from build123d import *

# Parameters (mm, degrees)
SKETCH1_W           = 167.5
SKETCH1_H           = 50
BOSS_EXTRUDE1_DEPTH = 5
BOSS_EXTRUDE2_REACH = 125.711
SKETCH3_R           = 2
CUT_EXTRUDE1_DEPTH  = 125.190739079
SKETCH6_R           = 1.947134786
BOSS_EXTRUDE7_DEPTH = 2.5
BOSS_EXTRUDE9_REACH = 133.18
SKETCH10_R          = 2
CUT_EXTRUDE3_DEPTH  = 132.180305898
FILLET2_R           = 5
SKETCH11_W          = 132.04
SKETCH11_H          = 9.88782449
CUT_EXTRUDE5_DEPTH  = 36


with BuildPart() as part:
    # Sketch1 → Boss-Extrude1 (new body)
    with BuildSketch(Plane.XY):
        Polygon((-83.75, 30), (-83.75, 55), (-89.745973018, 55), (-89.745973018, -55), (-83.75, -55), (-83.75, -30), (83.75, -30), (83.75, -55), (89.745973018, -55), (89.745973018, 55), (83.75, 55), (83.75, 30), align=None)
        Rectangle(SKETCH1_W, SKETCH1_H, mode=Mode.SUBTRACT)
    extrude(amount=BOSS_EXTRUDE1_DEPTH)

    # Boss-Extrude2: up to this face of the body (flat: up to its plane)
    boss_extrude2_end = Plane(part.part.faces().sort_by_distance((0, -30, 2.5))[0])
    # Sketch2 → Boss-Extrude2 (add, up to the picked face)
    with BuildSketch(Plane(origin=(0, 30, 0), x_dir=(1, 0, 0), z_dir=(0, 1, 0)), mode=Mode.PRIVATE) as boss_extrude2_sk1:
        with BuildLine():
            Line((-56.79, -5), (-63.79, -5))
            ThreePointArc((-63.79, -5), (-56.79, -12), (-49.79, -5))
            Line((-49.79, -5), (-56.79, -5))
        make_face()
    boss_extrude2_tool1 = split(extrude(boss_extrude2_sk1.sketch, amount=-BOSS_EXTRUDE2_REACH, mode=Mode.PRIVATE), bisect_by=boss_extrude2_end, keep=Keep.BOTH, mode=Mode.PRIVATE)
    # Sketch2 → Boss-Extrude2 (add, up to the picked face)
    with BuildSketch(Plane(origin=(0, 30, 0), x_dir=(1, 0, 0), z_dir=(0, 1, 0)), mode=Mode.PRIVATE) as boss_extrude2_sk2:
        Polygon((-63.79, 0), (-63.79, -5), (-56.79, -5), (-49.79, -5), (-49.79, 0), align=None)
    boss_extrude2_tool2 = split(extrude(boss_extrude2_sk2.sketch, amount=-BOSS_EXTRUDE2_REACH, mode=Mode.PRIVATE), bisect_by=boss_extrude2_end, keep=Keep.BOTH, mode=Mode.PRIVATE)
    add(boss_extrude2_tool1.solids().sort_by(Axis((-56.79, 30, 7.970892), (0, -1, 0)))[0])
    add(boss_extrude2_tool2.solids().sort_by(Axis((-56.79, 30, 2.5), (0, -1, 0)))[0])

    # Sketch3 → Cut-Extrude1 (cut, through all)
    with BuildSketch(Plane(origin=(0, 30, 0), x_dir=(1, 0, 0), z_dir=(0, 1, 0))):
        with Locations(Location((-56.79, -5, 0), (0, 0, 270))):
            Circle(SKETCH3_R)
    extrude(amount=-CUT_EXTRUDE1_DEPTH, mode=Mode.SUBTRACT)



with BuildPart() as body_2:
    # Sketch6 → Revolve2 (revolve)
    with BuildSketch(Plane(origin=(0, 0, 0), x_dir=(1, 0, 0), z_dir=(0, 1, 0))):
        with Locations((-97.245973018, -1.947134786)):
            Circle(SKETCH6_R)
    revolve(axis=Axis((-94.745973018, 0, 0), (0, 0, 1)))


with BuildPart() as part_1:
    add(part.part)

    add(body_2.part)  # Boss-Extrude7 merges body 2
    # Sketch9 → Boss-Extrude7 (add, symmetric)
    with BuildSketch(Plane(origin=(0, 0, 0), x_dir=(1, 0, 0), z_dir=(0, 1, 0))):
        Polygon((-92.245973018, 0), (-89.745973018, 0), (-89.745973018, -5), align=None)
    extrude(amount=BOSS_EXTRUDE7_DEPTH, both=True)

    # Boss-Extrude9: up to this face of the body (flat: up to its plane)
    boss_extrude9_end = Plane(part_1.part.faces().sort_by_distance((-4.055234189, -30, 2.93205693))[0])
    # Sketch4 → Boss-Extrude9 (add, up to the picked face)
    with BuildSketch(Plane(origin=(0, 30, 0), x_dir=(1, 0, 0), z_dir=(0, 1, 0)), mode=Mode.PRIVATE) as boss_extrude9_sk1:
        with BuildLine():
            Line((68.25, 0), (68.25, -5))
            ThreePointArc((68.25, -5), (61.25, -12), (54.25, -5))
            Line((54.25, -5), (54.25, 0))
            Line((54.25, 0), (68.25, 0))
        make_face()
    boss_extrude9_tool1 = split(extrude(boss_extrude9_sk1.sketch, amount=-BOSS_EXTRUDE9_REACH, mode=Mode.PRIVATE), bisect_by=boss_extrude9_end, keep=Keep.BOTH, mode=Mode.PRIVATE)
    add(boss_extrude9_tool1.solids().sort_by(Axis((61.25, 30, 5.365156), (0, -1, 0)))[0])

    # Sketch10 → Cut-Extrude3 (cut, through all)
    with BuildSketch(Plane(origin=(0, 30, 0), x_dir=(1, 0, 0), z_dir=(0, 1, 0))):
        with Locations(Location((61.25, -5, 0), (0, 0, 270))):
            Circle(SKETCH10_R)
    extrude(amount=-CUT_EXTRUDE3_DEPTH, mode=Mode.SUBTRACT)

    # Fillet2
    fillet2_edges = [part_1.edges().sort_by_distance(p)[0] for p in [
        (89.745973018, -55, 2.5),
        (89.745973018, 55, 2.5),
        (-89.745973018, 55, 2.5),
        (-89.745973018, -55, 2.5),
    ]]
    fillet(fillet2_edges, radius=FILLET2_R)

    # Sketch11 → Cut-Extrude5 (cut)
    with BuildSketch(Plane(origin=(0, 0, 0), x_dir=(-1, 0, 0), z_dir=(0, 0, -1))):
        with Locations((-2.23, 0)):
            Rectangle(SKETCH11_W, SKETCH11_H)
    extrude(amount=-CUT_EXTRUDE5_DEPTH, mode=Mode.SUBTRACT)


solid = part_1.part
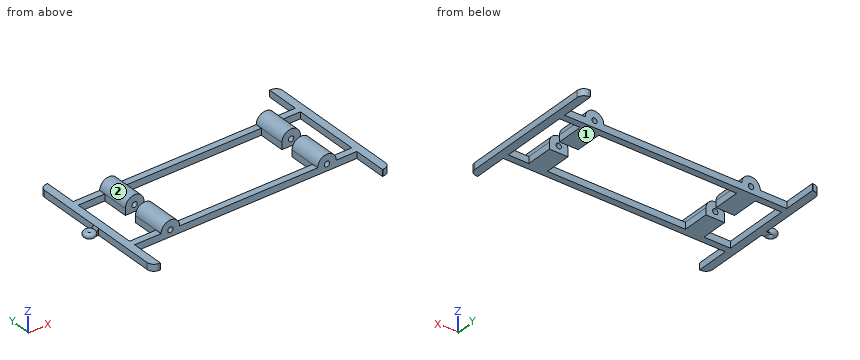
Work out the finished part from the listing and answer in its coordinate system (mm). Face numbers are marked on the shaded views. Round coordinates to 2 decimals unless told otherwise and drop trailing zeros. Write each loop counter-clockwise with the first axis right and the second up, starting at its lowest first coordinate (ties: lowest second). Pieces come first, ordered by that corner, then holes. Notation, with made-up numbers: (-7, 33) - (1, 33) arc R29 ccw to (1, 65) - close; hole circle Ø6 at (84, 81). An arc over 180 degrees is marked (long way). Answer in a Markdown table with one row per item. Add a question column.
1. The mould has two halves that part along X. Classify the marked faces 1 and 2: +X half, -X half, draft (parallel to the pull), parting line (faces both ways), or undercut.
2. A cutting plane is placed at A-A, the plane y = 44.5. Determine the outline of the cut face in (x, z), and give its area (3 significant figures).
3. A cutting plane is placed at B-B, the plane x = 61.25. Determine the outline of the cut face in (y, z).
4. A cutting plane is placed at C-C, the plane z = 9.5. Determine the outline of the cut face in (x, y), and give its area (3 significant figures).
5. Given pin 1 (1.3 mm diameter, centred on x = -91.5, z = 3, fed in from +Y); pin 2 (2.5 mm diameter, centred on y = 13.5, z = 3.5, fed in from -X); pin 3 (1.5 mm diameter, centred on x = -69.5, z = 2.5, fed in from -Y); pin 4 (4 mm diameter, centred on y = -40, z = 7.5, fed in from -X), each flat-ended and moving along its own axis, determine where each tip first touches the part or whether it passes through.
6. Find the intervals of material crossed by line 1 along X through (y, z) = (-27, 5.25); line 2 along X through (y, z) = (-38.5, 1); line 3 along Y through (x, z) = (-74.5, 4.5), in increasing order. Write a range as from..to.
7. A cutting plane is placed at D-D, the plane x = -11. Determine the outline of the cut face in (y, z), and give its area (3 significant figures).
Worked out:
| question | item | result |
|---|---|---|
| 1 | face 1 | draft |
| 1 | face 2 | undercut |
| 2 | outline | (-89.75, 0) - (-83.75, 0) - (-83.75, 5) - (-89.75, 5) - close; (83.75, 0) - (89.75, 0) - (89.75, 5) - (83.75, 5) - close |
| 2 | area | 60.0 mm^2 |
| 3 | outline | (-30, 0) - (-4.94, 0) - (-4.94, 3) - (-30, 3) - close; (-30, 7) - (-4.94, 7) - (-4.94, 12) - (-30, 12) - close; (4.94, 0) - (30, 0) - (30, 3) - (4.94, 3) - close; (4.94, 7) - (30, 7) - (30, 12) - (4.94, 12) - close |
| 4 | outline | (-62.15, -30) - (-51.43, -30) - (-51.43, -4.94) - (-62.15, -4.94) - close; (-62.15, 4.94) - (-51.43, 4.94) - (-51.43, 30) - (-62.15, 30) - close; (55.89, -30) - (66.61, -30) - (66.61, -4.94) - (55.89, -4.94) - close; (55.89, 4.94) - (66.61, 4.94) - (66.61, 30) - (55.89, 30) - close |
| 4 | area | 1,070 mm^2 |
| 5 | pin 1 | y = 3.37 |
| 5 | pin 2 | x = -89.75 |
| 5 | pin 3 | y = -30 |
| 5 | pin 4 | through |
| 6 | line 1 | -63.79..-58.77, -54.81..-49.79, 54.25..59.27, 63.23..68.25 |
| 6 | line 2 | -89.75..-83.75, 83.75..89.75 |
| 6 | line 3 | -30..-25, 25..30 |
| 7 | outline | (-30, 0) - (-25, 0) - (-25, 5) - (-30, 5) - close; (25, 0) - (30, 0) - (30, 5) - (25, 5) - close |
| 7 | area | 50.0 mm^2 |
